Work out the finished part from the listing and answer in its coordinate system (mm). Face numbers are marked on the shaded views. A direction names the side the tool comes from. Coordinates: 2 decimals unless noted, no trailing zeros. Order: outer loops, then holes, each group sorted by start corner. A loop starts at its lowest first (then second) coordinate and runs counter-clockwise, first axis right, second up. Notation, with made-up numbers: M 9.5,59.25 L 41.5,59.25 A10 cw 41.5,65.25 Z; hole C -4.5,52.5 d6. An arc over 180 degrees is marked long. Use a Markdown table: item, result.
from build123d import *

# Parameters (mm, degrees)
SWEEP1_PROFILE_R               = 37.5
SKETCH3_R                      = 55
BOSS_EXTRUDE1_DEPTH            = 10
TAP_DRILL_FOR_10_32_TAP1_D     = 4.0386
TAP_DRILL_FOR_10_32_TAP1_DEPTH = 10
SKETCH11_R                     = 7
CUT_EXTRUDE1_DEPTH             = 5


with BuildPart() as part:
    # Sweep1: sweep along a path in Sketch1
    with BuildLine(Plane(origin=(0, 0, 0), x_dir=(1, 0, 0), z_dir=(0, 1, 0))) as sweep1_path:
        Line((0, 0), (-75, 0))
        ThreePointArc((-75, 0), (-110.355339059, 14.644660941), (-125, 50))
        Line((-125, 50), (-125, 125))
    # Sweep1 profile (on start of the path) → Sweep1 (sweep)
    with BuildSketch(Plane(origin=(0, 0, 0), x_dir=(0, 0, -1), z_dir=(-1, 0, 0))):
        Circle(SWEEP1_PROFILE_R)
    sweep(path=sweep1_path.line)

    # Sketch3 → Boss-Extrude1 (add)
    with BuildSketch(Plane(origin=(0, 0, -125), x_dir=(-1, 0, 0), z_dir=(0, 0, -1))):
        with Locations((125, 0)):
            Circle(SKETCH3_R)
    extrude(amount=-BOSS_EXTRUDE1_DEPTH)

    # Tap Drill for #10-32 Tap1
    with Locations(Plane.XY.offset(-115)):
        with Locations((-148.75, 41.13620668), (-172.5, 0), (-148.75, -41.13620668), (-101.25, -41.13620668), (-77.5, 0), (-101.25, 41.13620668)):
            Hole(TAP_DRILL_FOR_10_32_TAP1_D / 2, depth=TAP_DRILL_FOR_10_32_TAP1_DEPTH)

    # Sketch11 → Cut-Extrude1 (cut)
    with BuildSketch(Plane(origin=(0, 0, -125), x_dir=(-1, 0, 0), z_dir=(0, 0, -1))):
        with Locations((146.817216858, 16.740939298)):
            Circle(SKETCH11_R)
        with Locations((122.414911455, 27.378227065)):
            Circle(SKETCH11_R)
        with Locations((100.434896061, 12.361458995)):
            Circle(SKETCH11_R)
        with Locations((101.47297262, -14.238292828)):
            Circle(SKETCH11_R)
        with Locations((124.556438483, -27.496422552)):
            Circle(SKETCH11_R)
        with Locations((148.055532132, -14.989744431)):
            Circle(SKETCH11_R)
    extrude(amount=-CUT_EXTRUDE1_DEPTH, mode=Mode.SUBTRACT)


solid = part.part
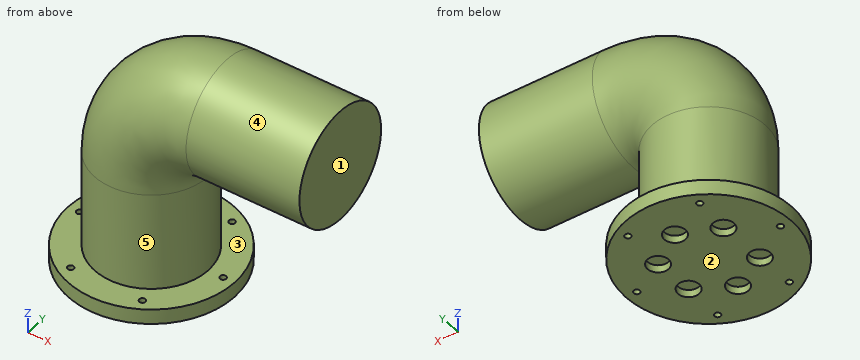
(1) Given P1, Ø4, axis at y = -26, z = -48.5, coming from the -X side; P2, Ø1, axis at y = 24.5, z = -50, coming from the +X side; P3, Ø5.5, axis at x = -148.75, y = -41.14, coming from the +Z side; P4, Ø3, axis at x = -148.75, y = 41.14, coming from the -Z side, each flat-ended and moving along its own axis, determine where each tip first touches the part or whether it passes through.
Conclusion:
| item | result |
|---|---|
| P1 | x = -153.8 |
| P2 | x = -96.19 |
| P3 | z = -115 |
| P4 | through |
(2) Straight lines are drawn through the part: L1, parallel to Z at x = -141, y = -40.5; L2, parallel to Z at x = -77, y = -11; L3, parallel to Z at x = -80.5, y = -17. For each, find the intervals that lie inside material, in ascending order.
Conclusion:
| item | result |
|---|---|
| L1 | -125 to -115 |
| L2 | -125 to -115, -35.99 to 35.83 |
| L3 | -125 to -115, -34.36 to 33.24 |
(3) A cutting plane is placed at C-C (z = -82). Determine the outline of the cut face in (x, y), then the cut area to 3 significant figures.
Conclusion:
| item | result |
|---|---|
| outline | C -125,0 d75 |
| area | 4,420 mm2 |
(4) Determine the mould class of the marked faces 1, 2 and 3 for opening direction Z: pulls with the +Z half, pulls with the -Z half, needs draft (parallel to the pull), parting line crosses it, or undercut.
Conclusion:
| item | result |
|---|---|
| face 1 | needs draft |
| face 2 | pulls with the -Z half |
| face 3 | undercut |
(5) A cutting plane is placed at B-B (x = -52). Determine the outline of the cut face in (y, z).
Conclusion:
| item | result |
|---|---|
| outline | C 0,0 d75 |
(6) Which of the six approach directions +Z, -Z, +X, -X, +Y, -Y give full straight-line access (tool end or side, diameter ignored) to the marked faces 4 and 5?
Conclusion:
| item | result |
|---|---|
| face 4 | +X |
| face 5 | none |
(7) A cutting plane is placed at A-A (x = -72.5). Determine the outline of the cut face in (y, z).
Conclusion:
| item | result |
|---|---|
| outline | C 0,0 d75; M -16.39,-125 L 16.39,-125 L 16.39,-115 L -16.39,-115 Z |
